from build123d import *

# Parameters (mm, degrees)
F0_W     = 76.2
F0_H     = 25.4
F1_DEPTH = 31.75
F3_DEPTH = 25.4


with BuildPart() as f1:
    # F0 (on Top) → F1 (new body)
    with BuildSketch(Plane.XY):
        Rectangle(F0_W, F0_H)
    extrude(amount=F1_DEPTH)

    # F2 (on face) → F3 (cut)
    with BuildSketch(Plane.XY.offset(31.75)):
        with BuildLine():
            Line((-7.62, 0), (0, 0))
            Line((0, 0), (6.096, 0))
            ThreePointArc((6.096, 0), (-0.762, 6.858), (-7.62, 0))
        make_face()
        with BuildLine():
            Line((6.096, 0), (0, 0))
            Line((0, 0), (-7.62, 0))
            ThreePointArc((-7.62, 0), (-0.762, -6.858), (6.096, 0))
        make_face()
        with BuildLine():
            ThreePointArc((31.366032, 0), (29.334032, 2.032), (27.302032, 0))
            Line((27.302032, 0), (31.366032, 0))
        make_face()
        with BuildLine():
            Line((31.366032, 0), (27.302032, 0))
            ThreePointArc((27.302032, 0), (29.334032, -2.032), (31.366032, 0))
        make_face()
        with BuildLine():
            ThreePointArc((19.304, 0), (17.018, 2.286), (14.732, 0))
            Line((14.732, 0), (19.304, 0))
        make_face()
        with BuildLine():
            Line((19.304, 0), (14.732, 0))
            ThreePointArc((14.732, 0), (17.018, -2.286), (19.304, 0))
        make_face()
        with BuildLine():
            ThreePointArc((-30.48, 0), (-23.622, -6.858), (-16.764, 0))
            Line((-16.764, 0), (-30.48, 0))
        make_face()
        with BuildLine():
            Line((-30.48, 0), (-16.764, 0))
            ThreePointArc((-16.764, 0), (-23.622, 6.858), (-30.48, 0))
        make_face()
    extrude(amount=-F3_DEPTH, mode=Mode.SUBTRACT)


solid = f1.part
For this review, take the finished solid that the model builds, in its own axes (mm). A direction names the side the tool comes from. Give positions to 0.01 mm unless a question says otherwise; leave off trailing zeros. Loops run counter-clockwise (first coordinate to the right, second up) from the corner with the lowest first, then second, coordinate; pieces in that order, holes last.
Item 1: Tool access review of faces 1 (the flat face through (8, 0, 31.75)), 2 (the cylindrical face through (6.09, -0.3, 19.23)): name each direction out of +Z, -Z, +X, -X, +Y, -Y from which nothing blocks a thin tool from reaching the whole face with its end or side.
Item 2: Take a section at B-B, the plane y = 0. State the section outline as (x, z) points, and give its area (3 significant figures).
Item 3: Insertion check: pin 1 (11 mm diameter, centred on x = -23.622, y = 0, fed in from +Z). The pin has a flat end and moves straight along its axis. Give the tip position at first contact, or say it passes through.
Item 4: For line 1 along X through (y, z) = (2.5, 17); line 2 along X through (y, z) = (5.5, 21.5); line 3 along Y through (x, z) = (-6, 12), list the stretches that pass through material, from the lowest coordinate up.
Item 5: Take a section at D-D, the plane x = -28.5. State the section outline as (y, z) points.
Item 6: Take a section at A-A, the plane z = 15. State the section outline as (x, y) points.
Item 7: Take a section at C-C, the plane x = 17. State the section outline as (y, z) points.
Item 8: Draft analysis for pull direction Y (two halves, no side actions). For faces 3 (the flat face through (-1, 0, 6.35)), 4 (the flat face through (-1, -12.7, 16)), 5 (the flat face through (17, 0, 6.35)), 6 (the flat face through (38.1, 0, 16)), state which applies: +Y half, -Y half, draft (parallel to the pull), parting line (faces both ways), or undercut.
Calculated:
1. face 1: +Z, +X, -X, +Y, -Y
1. face 2: +Z
2. outline: (-38.1, 0) - (38.1, 0) - (38.1, 31.75) - (31.37, 31.75) - (31.37, 6.35) - (27.3, 6.35) - (27.3, 31.75) - (19.3, 31.75) - (19.3, 6.35) - (14.73, 6.35) - (14.73, 31.75) - (6.1, 31.75) - (6.1, 6.35) - (-7.62, 6.35) - (-7.62, 31.75) - (-16.76, 31.75) - (-16.76, 6.35) - (-30.48, 6.35) - (-30.48, 31.75) - (-38.1, 31.75) - close
2. area: 1,500 mm2
3. pin 1: stops at z = 6.35
4. line 1: x = -38.1 to -30.01, -17.24 to -7.15, 5.62 to 38.1
4. line 2: x = -38.1 to -27.72, -19.53 to -4.86, 3.33 to 38.1
4. line 3: y = -12.7 to -4.43, 4.43 to 12.7
5. outline: (-12.7, 0) - (12.7, 0) - (12.7, 31.75) - (4.82, 31.75) - (4.82, 6.35) - (-4.82, 6.35) - (-4.82, 31.75) - (-12.7, 31.75) - close
6. outline: (-38.1, -12.7) - (38.1, -12.7) - (38.1, 12.7) - (-38.1, 12.7) - close; hole circle Ø13.72 at (-23.62, 0); hole circle Ø13.72 at (-0.76, 0); hole circle Ø4.57 at (17.02, 0); hole circle Ø4.06 at (29.33, 0)
7. outline: (-12.7, 0) - (12.7, 0) - (12.7, 31.75) - (2.29, 31.75) - (2.29, 6.35) - (-2.29, 6.35) - (-2.29, 31.75) - (-12.7, 31.75) - close
8. face 3: undercut
8. face 4: -Y half
8. face 5: undercut
8. face 6: draft
